```python
from build123d import *

# Parameters (mm, degrees)
F0_R     = 38.1
F0_R_2   = 8.763
F1_DEPTH = 25.4
F2_R     = 3.302
F3_DEPTH = 30.48
F4_R     = 15.24
F4_R_2   = 8.763
F5_DEPTH = 17.78
F6_R     = 18.082851
F6_R_2   = 8.763
F7_DEPTH = 5.08


with BuildPart() as f1:
    # F0 (on Front) → F1 (new body)
    with BuildSketch(Plane.XZ):
        Circle(F0_R)
        Circle(F0_R_2, mode=Mode.SUBTRACT)
    extrude(amount=F1_DEPTH)

    # F2 (on face) → F3 (cut)
    with BuildSketch(Plane(origin=(0, 0, 0), x_dir=(-1, 0, 0), z_dir=(0, 1, 0))):
        with Locations((0, 32.246636)):
            Circle(F2_R)
        with Locations((-9.964759, 30.668374)):
            Circle(F2_R)
        with Locations((-18.954097, 26.088077)):
            Circle(F2_R)
        with Locations((-26.088077, 18.954097)):
            Circle(F2_R)
        with Locations((-30.668374, 9.964759)):
            Circle(F2_R)
        with Locations((-32.246636, 0)):
            Circle(F2_R)
        with Locations((-30.668374, -9.964759)):
            Circle(F2_R)
        with Locations((-26.088077, -18.954097)):
            Circle(F2_R)
        with Locations((-18.954097, -26.088077)):
            Circle(F2_R)
        with Locations((-9.964759, -30.668374)):
            Circle(F2_R)
        with Locations((0, -32.246636)):
            Circle(F2_R)
        with Locations((9.964759, -30.668374)):
            Circle(F2_R)
        with Locations((18.954097, -26.088077)):
            Circle(F2_R)
        with Locations((26.088077, -18.954097)):
            Circle(F2_R)
        with Locations((30.668374, -9.964759)):
            Circle(F2_R)
        with Locations((32.246636, 0)):
            Circle(F2_R)
        with Locations((30.668374, 9.964759)):
            Circle(F2_R)
        with Locations((26.088077, 18.954097)):
            Circle(F2_R)
        with Locations((18.954097, 26.088077)):
            Circle(F2_R)
        with Locations((9.964759, 30.668374)):
            Circle(F2_R)
    extrude(amount=-F3_DEPTH, mode=Mode.SUBTRACT)

    # F4 (on face) → F5 (join)
    with BuildSketch(Plane.XZ.offset(25.4)):
        Circle(F4_R)
        Circle(F4_R_2, mode=Mode.SUBTRACT)
    extrude(amount=F5_DEPTH)

    # F6 (on face) → F7 (join)
    with BuildSketch(Plane(origin=(0, 0, 0), x_dir=(-1, 0, 0), z_dir=(0, 1, 0))):
        Circle(F6_R)
        Circle(F6_R_2, mode=Mode.SUBTRACT)
    extrude(amount=F7_DEPTH)


solid = f1.part
```
Here's how the part is built. I have some questions about the finished solid (model axes, mm). A direction names the side the tool comes from. Coordinates: 2 decimals unless noted, no trailing zeros. Write each loop counter-clockwise with the first axis right and the second up, starting at its lowest first coordinate (ties: lowest second). Pieces come first, ordered by that corner, then holes. Notation, with made-up numbers: M 4,26 L 39,26 A8 cw 39,32 Z; hole C 61,21 d3. An arc over 180 degrees is marked long. Answer as CSV lines item,"result". Start each with the question number.
Q1. Suppose I cut it at A-A, the plane x = 0. List the corners of the cut face in (y, z) for me, then the cut area to 3 significant figures.
Q2. Suppose I cut it at B-B, the plane z = 0. List the corners of the cut face in (x, y) for me, then the cut area to 3 significant figures.
Q3. Suppose I cut it at C-C, the plane y = -31. List the corners of the cut face in (x, z) for me, then the cut area to 3 significant figures.
Q4. Suppose I cut it at D-D, the plane y = -23. State how many separate pieces and enclosed holes the cut face has, then the cut area to 3 significant figures.
Q5. For faces 5 (the cylindrical face through (-29.138, -12.522, -20.219)), 6 (the flat face through (16, -25.4, 1)), which set-ups out of +Z, -Z, +X, -X, +Y, -Y let a thin tool reach every point of the face, with its end or its side?
Q6. I need wall thicknesses on probe 1 along X at (y, z) = (-15, 9); probe 2 along Z at (x, y) = (30, -10); probe 3 along X at (y, z) = (-9, 23.5). Which ranges of each line are inside material? Lowest first, please. Write a range as [from, to].
Q7. Will these pins go through, and if not, where does the flat tip stop? pin 1 Ø5.5 at (x, z) = (-18.95, -26.09) entering from +Y; pin 2 Ø10.5 at (x, z) = (18.95, -26.09) entering from -Y; pin 3 Ø8.5 at (x, z) = (26.09, -18.95) entering from +Y; pin 4 Ø4 at (x, y) = (2.5, -21.5) entering from -Z.
Q8. If we mould it in two halves opening along Z, with no side actions, what happens to faces 1 (the cylindrical face through (-16.334, -12.522, -28.097)), 2 (the flat face through (4, 5.08, -8)), 3 (the cylindrical face through (-9.72, 2.5, 15.25)), 4 (the cylindrical face through (-13.114, -12.522, -29.677))? For each: pulls with the +Z half, pulls with the -Z half, needs draft (parallel to the pull), parting line crosses it, or undercut.
Entries:
1,outline,"M -43.18,-15.24 L -25.4,-15.24 L -25.4,-28.94 L 0,-28.94 L 0,-18.08 L 5.08,-18.08 L 5.08,-8.76 L -43.18,-8.76 Z; M -43.18,8.76 L 5.08,8.76 L 5.08,18.08 L 0,18.08 L 0,28.94 L -25.4,28.94 L -25.4,15.24 L -43.18,15.24 Z; M -25.4,-38.1 L 0,-38.1 L 0,-35.55 L -25.4,-35.55 Z; M -25.4,35.55 L 0,35.55 L 0,38.1 L -25.4,38.1 Z"
1,area,"1,480 mm²"
2,outline,"M -38.1,-25.4 L -35.55,-25.4 L -35.55,0 L -38.1,0 Z; M -28.94,-25.4 L -15.24,-25.4 L -15.24,-43.18 L -8.76,-43.18 L -8.76,5.08 L -18.08,5.08 L -18.08,0 L -28.94,0 Z; M 8.76,-43.18 L 15.24,-43.18 L 15.24,-25.4 L 28.94,-25.4 L 28.94,0 L 18.08,0 L 18.08,5.08 L 8.76,5.08 Z; M 35.55,-25.4 L 38.1,-25.4 L 38.1,0 L 35.55,0 Z"
2,area,"1,480 mm²"
3,outline,"C 0,0 d30.48; hole C 0,0 d17.53"
3,area,"488 mm²"
4,separate pieces,"1"
4,enclosed holes,"21"
4,area,"3,630 mm²"
5,face 5,"+Y, -Y"
5,face 6,"-Y"
6,probe 1,"x = [-37.02, -33.83], [-27.51, 27.51], [33.83, 37.02]"
6,probe 2,"z = [-23.49, -13.2], [-6.73, -2.42], [2.42, 6.73], [13.2, 23.49]"
6,probe 3,"x = [-29.99, -21], [-16.9, 16.9], [21, 29.99]"
7,pin 1,"passes through"
7,pin 2,"stops at y = -25.4"
7,pin 3,"stops at y = 0"
7,pin 4,"stops at z = -38.1"
8,face 1,"undercut"
8,face 2,"needs draft"
8,face 3,"parting line crosses it"
8,face 4,"undercut"
